Geometry: final body of the model. Coordinates: model frame, mm. A direction names the side the tool comes from. Coordinates: 2 decimals unless noted, no trailing zeros. Order: outer loops, then holes, each group sorted by start corner. A loop starts at its lowest first (then second) coordinate and runs counter-clockwise, first axis right, second up. Notation, with made-up numbers: (20.25, 63) - (58.25, 63) arc R26 cw to (58.25, 82) - close; hole circle Ø3 at (33.5, -32.5). An arc over 180 degrees is marked (long way). Use one line per item in the form item = value. Start each with the question number.
```python
from build123d import *

# Parameters (mm, degrees)
SKETCH_1_R      = 27.6
SKETCH_1_R_2    = 1.7
EXTRUDE_1_DEPTH = 3
EXTRUDE_START   = -6
SKETCH_2_R      = 29.5
SKETCH_2_R_2    = 27.6
EXTRUDE_2_DEPTH = 6


with BuildPart() as part:
    # 草图1 → 凸台-拉伸1 (new body)
    with BuildSketch(Plane.XY):
        Circle(SKETCH_1_R)
        with Locations((-14.505925513, -8.375)):
            Circle(SKETCH_1_R_2, mode=Mode.SUBTRACT)
        with Locations((-14.505925513, 8.375)):
            Circle(SKETCH_1_R_2, mode=Mode.SUBTRACT)
        with Locations((0, 16.75)):
            Circle(SKETCH_1_R_2, mode=Mode.SUBTRACT)
        with Locations((14.505925513, 8.375)):
            Circle(SKETCH_1_R_2, mode=Mode.SUBTRACT)
        with Locations((14.505925513, -8.375)):
            Circle(SKETCH_1_R_2, mode=Mode.SUBTRACT)
        with Locations((0, -16.75)):
            Circle(SKETCH_1_R_2, mode=Mode.SUBTRACT)
    extrude(amount=EXTRUDE_1_DEPTH)

    # 草图2 → 凸台-拉伸2 (add)
    with BuildSketch(Plane.XY.offset(3).offset(EXTRUDE_START)):
        Circle(SKETCH_2_R)
        Circle(SKETCH_2_R_2, mode=Mode.SUBTRACT)
    extrude(amount=EXTRUDE_2_DEPTH)


solid = part.part
```
(1) Cut plane D-D on y = -16.75. Return the cut outline in (x, z).
(2) Cut plane C-C on z = 1.2. Return the cut outline in (x, y) (3 decimals), plus the area to 3 significant figures.
(3) Draft query along Y for faces 3 (the flat face through (20, -20, -3)), 4 (the cylindrical face through (28.14, 8.86, -0.04)), 5 (the cylindrical face through (-12.936, -9.026, 1.479)). Return one class per face: released by +Y, released by -Y, zero draft, split by the parting line, or undercut.
(4) Cut plane B-B on y = 0. Return the cut outline in (x, z), plus the area to 3 significant figures.
(5) Contact query for flat-ended pins moving along their axis: pin 1 Ø3 at (y, z) = (14.5, 1.5) entering from +X; pin 2 Ø5.5 at (x, y) = (14.51, -8.38) entering from -Z; pin 3 Ø1.5 at (x, z) = (-19, -1.5) entering from +Y. Output: stop coordinate, or through.
(6) Material intervals for L1, parallel to Y at x = 0, z = 1.25; L2, parallel to Y at x = 1.5, z = 0.1; L3, parallel to Z at x = 10.5, y = 20.5, sorted ascending. Write a range as from..to.
(7) Set-up query: faces 1 (the cylindrical face through (-3.593, 27.365, -1.521)), 2 (the cylindrical face through (-12.936, 7.724, 1.479)). Return all of +Z, -Z, +X, -X, +Y, -Y with unobstructed straight access to the full face (end or side cutting, diameter ignored); none if empty.
(8) Cut plane A-A on x = 0. Return the cut outline in (y, z), plus the area to 3 significant figures.
Check sheet entries:
q1.outline = (-24.28, -3) - (-21.94, -3) - (-21.94, 0) - (-1.7, 0) - (-1.7, 3) - (-24.28, 3) - close; (1.7, 0) - (21.94, 0) - (21.94, -3) - (24.28, -3) - (24.28, 3) - (1.7, 3) - close
q2.outline = circle Ø59 at (0, 0); hole circle Ø3.4 at (-14.506, -8.375); hole circle Ø3.4 at (-14.506, 8.375); hole circle Ø3.4 at (0, -16.75); hole circle Ø3.4 at (0, 16.75); hole circle Ø3.4 at (14.506, -8.375); hole circle Ø3.4 at (14.506, 8.375)
q2.area = 2,680 mm^2
q3.face_3 = zero draft
q3.face_4 = split by the parting line
q3.face_5 = undercut
q4.outline = (-29.5, -3) - (-27.6, -3) - (-27.6, 0) - (27.6, 0) - (27.6, -3) - (29.5, -3) - (29.5, 3) - (-29.5, 3) - close
q4.area = 188 mm^2
q5.pin_1 = 26.48
q5.pin_2 = 0
q5.pin_3 = 23.18
q6.L1 = -29.5..-18.45, -15.05..15.05, 18.45..29.5
q6.L2 = -29.46..-17.55, -15.95..15.95, 17.55..29.46
q6.L3 = 0..3
q7.face_1 = -Z
q7.face_2 = +Z, -Z
q8.outline = (-29.5, -3) - (-27.6, -3) - (-27.6, 0) - (-18.45, 0) - (-18.45, 3) - (-29.5, 3) - close; (-15.05, 0) - (15.05, 0) - (15.05, 3) - (-15.05, 3) - close; (18.45, 0) - (27.6, 0) - (27.6, -3) - (29.5, -3) - (29.5, 3) - (18.45, 3) - close
q8.area = 168 mm^2
